from build123d import *

# Parameters (mm, degrees)
SKETCH4_R           = 2
SKETCH4_R_2         = 2.85
SKETCH4_W           = 22
SKETCH4_H           = 32
BOSS_EXTRUDE1_DEPTH = 5
FILLET1_R           = 5
CHAMFER1_SIZE       = 0.5


with BuildPart() as part:
    # Sketch4 → Boss-Extrude1 (new, symmetric)
    with BuildSketch(Plane.XY):
        with BuildLine():
            ThreePointArc((69.282032303, -10), (0, 70), (-69.282032303, -10))
            Line((-69.282032303, -10), (-35, 9.792740578))
            Line((-35, 9.792740578), (-35, -55))
            Line((-35, -55), (-35, -65))
            Line((-35, -65), (-15, -105))
            Line((-15, -105), (-7.5, -105))
            Line((-7.5, -105), (-7.5, -90))
            Line((-7.5, -90), (7.5, -90))
            Line((7.5, -90), (7.5, -105))
            Line((7.5, -105), (15, -105))
            Line((15, -105), (35, -65))
            Line((35, -65), (35, 9.792740578))
            Line((35, 9.792740578), (69.282032303, -10))
        make_face()
        with Locations((-8.75, -87)):
            Circle(SKETCH4_R, mode=Mode.SUBTRACT)
        with Locations((-25, -45)):
            Circle(SKETCH4_R_2, mode=Mode.SUBTRACT)
        with Locations((8.75, -87)):
            Circle(SKETCH4_R, mode=Mode.SUBTRACT)
        with Locations((25, -45)):
            Circle(SKETCH4_R_2, mode=Mode.SUBTRACT)
        with BuildLine():
            Line((25, -32.5), (-25, -32.5))
            ThreePointArc((-25, -32.5), (-27.5, -30), (-25, -27.5))
            Line((-25, -27.5), (25, -27.5))
            ThreePointArc((25, -27.5), (27.5, -30), (25, -32.5))
        make_face(mode=Mode.SUBTRACT)
        with Locations((-18, 0)):
            Circle(SKETCH4_R_2, mode=Mode.SUBTRACT)
        with BuildLine():
            Line((-30, 24.226497308), (-59.572090597, 7.153042841))
            ThreePointArc((-59.572090597, 7.153042841), (-50.077338732, 33.04935923), (-30, 51.961524227))
            Line((-30, 51.961524227), (-30, 24.226497308))
        make_face(mode=Mode.SUBTRACT)
        with Locations((-22, 30)):
            Circle(SKETCH4_R_2, mode=Mode.SUBTRACT)
        with Locations((0, 46)):
            Rectangle(SKETCH4_W, SKETCH4_H, mode=Mode.SUBTRACT)
        with Locations((18, 0)):
            Circle(SKETCH4_R_2, mode=Mode.SUBTRACT)
        with BuildLine():
            Line((25, 12.5), (-25, 12.5))
            ThreePointArc((-25, 12.5), (-27.5, 15), (-25, 17.5))
            Line((-25, 17.5), (25, 17.5))
            ThreePointArc((25, 17.5), (27.5, 15), (25, 12.5))
        make_face(mode=Mode.SUBTRACT)
        with Locations((22, 30)):
            Circle(SKETCH4_R_2, mode=Mode.SUBTRACT)
        with BuildLine():
            Line((59.572090597, 7.153042841), (30, 24.226497308))
            Line((30, 24.226497308), (30, 51.961524227))
            ThreePointArc((30, 51.961524227), (50.077338732, 33.04935923), (59.572090597, 7.153042841))
        make_face(mode=Mode.SUBTRACT)
    extrude(amount=BOSS_EXTRUDE1_DEPTH, both=True)

    # Fillet1
    # the kernel refuses this fillet: 5 mm, written as the material it adds along each edge
    with BuildSketch(Plane(origin=(59.572090597, 7.153042841, -5), x_dir=(-0.8660254037844397, 0.49999999999999806, 0), z_dir=(0, 0, 1))) as fillet1_piece_1:
        with BuildLine():
            CenterArc((11.332313176, -5), FILLET1_R, 90, 138.168098297)
            ThreePointArc((7.997575975, -8.725523829), (3.783101322, -4.560454399), (0, 0))
            Line((0, 0), (11.332313176, 0))
        make_face()
    extrude(amount=10)
    with BuildSketch(Plane(origin=(30, 24.226497308, 5), x_dir=(0, 1, 0), z_dir=(0, 0, -1))) as fillet1_piece_2:
        with BuildLine():
            CenterArc((FILLET1_R * 0.57735026919, FILLET1_R), FILLET1_R, 210, 60)
            Line((-FILLET1_R * 0.288675134595, FILLET1_R * 0.5), (0, 0))
            Line((0, 0), (FILLET1_R * 0.57735026919, 0))
        make_face()
    extrude(amount=10)
    with BuildSketch(Plane(origin=(30, 51.961524227, -5), x_dir=(0, -1, 0), z_dir=(0, 0, 1))) as fillet1_piece_3:
        with BuildLine():
            CenterArc((9.535117356, 5), FILLET1_R, 140.478803641, 129.521196359)
            ThreePointArc((5.678171277, 8.181818182), (2.669034839, 4.208924127), (0, 0))
            Line((0, 0), (9.535117356, 0))
        make_face()
    extrude(amount=10)
    with BuildSketch(Plane(origin=(-59.572090597, 7.153042841, 5), x_dir=(0.2165677144201491, 0.9762675991094004, 0), z_dir=(0, 0, -1))) as fillet1_piece_4:
        with BuildLine():
            CenterArc((11.343039457, 4.975618333), FILLET1_R, 137.492482071, 138.168098297)
            Line((7.657096034, 8.354053043), (0, 0))
            ThreePointArc((0, 0), (5.918107543, -0.29258), (11.836215086, 0))
        make_face()
    extrude(amount=10)
    with BuildSketch(Plane(origin=(-30, 24.226497308, -5), x_dir=(-0.8660254037844397, -0.49999999999999795, 0), z_dir=(0, 0, 1))) as fillet1_piece_5:
        with BuildLine():
            CenterArc((FILLET1_R * 0.57735026919, -FILLET1_R), FILLET1_R, 90, 60)
            Line((-FILLET1_R * 0.288675134595, -FILLET1_R * 0.5), (0, 0))
            Line((0, 0), (FILLET1_R * 0.57735026919, 0))
        make_face()
    extrude(amount=10)
    with BuildSketch(Plane(origin=(-30, 51.961524227, -5), x_dir=(-0.8215414898046486, -0.5701487354450225, 0), z_dir=(0, 0, 1))) as fillet1_piece_6:
        with BuildLine():
            CenterArc((9.544142552, 4.982750841), FILLET1_R, 145.239401821, 129.521196359)
            Line((5.436435103, 7.833494518), (0, 0))
            ThreePointArc((0, 0), (4.979552636, -0.206989911), (9.959105271, 0))
        make_face()
    extrude(amount=10)
    with BuildSketch(Plane(origin=(35, 9.792740578, -5), x_dir=(0.8660254037844399, -0.49999999999999795, 0), z_dir=(0, 0, 1)), Plane(origin=(-35, 9.792740578, -5), x_dir=(0, -1, 0), z_dir=(0, 0, 1))) as fillet1_piece_7:
        with BuildLine():
            CenterArc((FILLET1_R * 1.73205080757, -FILLET1_R), FILLET1_R, 90, 120)
            Line((FILLET1_R * 0.866025403784, -FILLET1_R * 1.5), (0, 0))
            Line((0, 0), (FILLET1_R * 1.73205080757, 0))
        make_face()
    extrude(amount=10)
    with BuildSketch(Plane(origin=(7.5, -90, 5), x_dir=(0, -1, 0), z_dir=(0, 0, -1)), Plane(origin=(-7.5, -90, 5), x_dir=(1, 0, 0), z_dir=(0, 0, -1))) as fillet1_piece_8:
        with BuildLine():
            CenterArc((FILLET1_R, FILLET1_R), FILLET1_R, 180, 90)
            Line((0, FILLET1_R), (0, 0))
            Line((0, 0), (FILLET1_R, 0))
        make_face()
    extrude(amount=10)
    # the kernel refuses this fillet: 5 mm, written as the material it takes off along each edge
    with BuildSketch(Plane(origin=(-69.282032303, -10, -25.386938297), x_dir=(-0.08496362878818808, 0.9963840533565073, 0), z_dir=(0, 0, 1))) as fillet1_2_piece_1:
        with BuildLine():
            CenterArc((7.863533343, -4.991510604), FILLET1_R, 86.660722685, 118.465343928)
            Line((3.33665476, -7.114567433), (0, 0))
            ThreePointArc((0, 0), (4.077387659, 0.118851542), (8.154775319, 0))
        make_face()
    extrude(amount=50.773876593, mode=Mode.SUBTRACT)
    with BuildSketch(Plane(origin=(69.282032303, -10, -25.386938297), x_dir=(-0.8660254037844397, 0.4999999999999982, 0), z_dir=(0, 0, 1))) as fillet1_2_piece_2:
        with BuildLine():
            CenterArc((7.858138122, -5), FILLET1_R, 90, 118.465343928)
            ThreePointArc((3.462610285, -7.383135547), (1.623699843, -3.742033489), (0, 0))
            Line((0, 0), (7.858138122, 0))
        make_face()
    extrude(amount=50.773876593, mode=Mode.SUBTRACT)
    with BuildSketch(Plane(origin=(15, -105, -12.725424859), x_dir=(-1, 0, 0), z_dir=(0, 0, 1)), Plane(origin=(-15, -105, -12.725424859), x_dir=(-0.4472135954999598, 0.894427190999915, 0), z_dir=(0, 0, 1))) as fillet1_2_piece_3:
        with BuildLine():
            CenterArc((FILLET1_R * 0.61803398875, -FILLET1_R), FILLET1_R, 90, 63.434948823)
            Line((-FILLET1_R * 0.27639320225, -FILLET1_R * 0.5527864045), (0, 0))
            Line((0, 0), (FILLET1_R * 0.61803398875, 0))
        make_face()
    extrude(amount=25.450849719, mode=Mode.SUBTRACT)
    with BuildSketch(Plane(origin=(7.5, -105, -17.5), x_dir=(0, 1, 0), z_dir=(0, 0, 1))) as fillet1_2_piece_4:
        with BuildLine():
            CenterArc((FILLET1_R, -FILLET1_R), FILLET1_R, 90, 90)
            Line((0, -FILLET1_R), (0, 0))
            Line((0, 0), (FILLET1_R, 0))
        make_face()
    extrude(amount=35, mode=Mode.SUBTRACT)
    with BuildSketch(Plane(origin=(-7.5, -105, 17.5), x_dir=(-1, 0, 0), z_dir=(0, 0, -1))) as fillet1_2_piece_5:
        with BuildLine():
            CenterArc((FILLET1_R, FILLET1_R), FILLET1_R, 180, 90)
            Line((0, FILLET1_R), (0, 0))
            Line((0, 0), (FILLET1_R, 0))
        make_face()
    extrude(amount=35, mode=Mode.SUBTRACT)

    # Chamfer1
    chamfer1_edges = [part.edges().sort_by_distance(p)[0] for p in [
        (22.15, -45, 5),
        (19.15, 30, 5),
        (15.15, 0, 5),
        (6.75, -87, 5),
        (-10.75, -87, 5),
        (-24.85, 30, 5),
        (-20.85, 0, 5),
        (-27.85, -45, 5),
    ]]
    chamfer(chamfer1_edges, length=CHAMFER1_SIZE)


solid = part.part
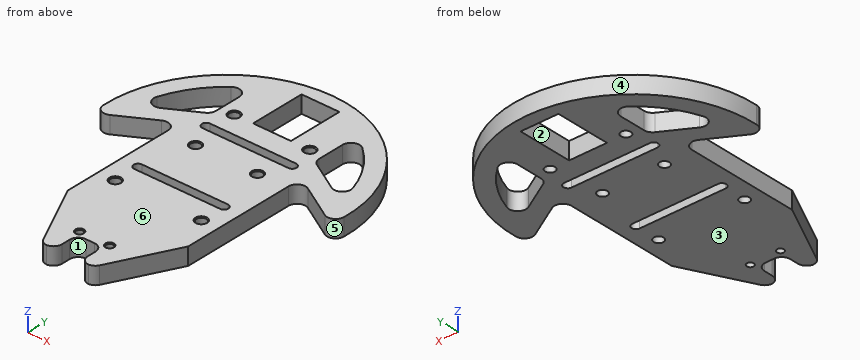
Source: CAD feature listing. Evaluate the final solid. Frame: model axes, mm. Face numbers are marked on the shaded views. A direction names the side the tool comes from. Coordinates: 2 decimals unless noted, no trailing zeros. Write each loop counter-clockwise with the first axis right and the second up, starting at its lowest first coordinate (ties: lowest second). Pieces come first, ordered by that corner, then holes. Notation, with made-up numbers: M 87.25,-18.75 L 94.25,-18.75 A20 ccw 94.25,0.25 Z; hole C -39,63.25 d1. An arc over 180 degrees is marked long. Use a Markdown table: item, result.
1) Ray query, L1, parallel to Y at x = -15, z = -1; L2, parallel to Y at x = -18, z = 1; L3, parallel to X at y = 34, z = -2.25. Return the intervals inside material, ascending.
Conclusion:
| item | result |
|---|---|
| L1 | y = -103.93 to -32.5, -27.5 to 12.5, 17.5 to 68.37 |
| L2 | y = -99 to -32.5, -27.5 to -2.85, 2.85 to 12.5, 17.5 to 67.65 |
| L3 | x = -61.19 to -49.44, -30 to -11, 11 to 30, 49.44 to 61.19 |
2) Section A-A, the plane y = -87. Output: boundary loops of the cut face in (x, z).
Conclusion:
| item | result |
|---|---|
| outline | M -24,-5 L -10.75,-5 L -10.75,4.5 L -11.25,5 L -24,5 Z; M -6.75,-5 L 6.75,-5 L 6.75,4.5 L 6.25,5 L -6.25,5 L -6.75,4.5 Z; M 10.75,-5 L 24,-5 L 24,5 L 11.25,5 L 10.75,4.5 Z |
3) Section D-D, the plane x = -45. Output: boundary loops of the cut face in (y, z).
Conclusion:
| item | result |
|---|---|
| outline | M 4.02,-5 L 15.57,-5 L 15.57,5 L 4.02,5 Z; M 39.69,-5 L 53.62,-5 L 53.62,5 L 39.69,5 Z |
4) Section B-B, the plane x = 0. Output: boundary loops of the cut face in (y, z).
Conclusion:
| item | result |
|---|---|
| outline | M -90,-5 L -32.5,-5 L -32.5,5 L -90,5 Z; M -27.5,-5 L 12.5,-5 L 12.5,5 L -27.5,5 Z; M 17.5,-5 L 30,-5 L 30,5 L 17.5,5 Z; M 62,-5 L 70,-5 L 70,5 L 62,5 Z |
5) Reachability of the marked faces 1, 2 and 3 from +Z, -Z, +X, -X, +Y, -Y: full face, straight path, thin tool, end or side. Return the list, or none.
Conclusion:
| item | result |
|---|---|
| face 1 | +Z, -Z, -Y |
| face 2 | +Z, -Z |
| face 3 | -Z, +X, -X, +Y, -Y |
6) Mould query, pull axis X, two halves, no side actions, for the marked faces 4, 5 and 6. Classes: pulls with the +X half, pulls with the -X half, needs draft (parallel to the pull), parting line crosses it, or undercut.
Conclusion:
| item | result |
|---|---|
| face 4 | parting line crosses it |
| face 5 | undercut |
| face 6 | needs draft |
7) First-contact query: pin 1 Ø7.5 at (x, y) = (25, -45) entering from +Z; pin 2 Ø5 at (y, z) = (-23.5, 0.5) entering from +X; pin 3 Ø5.5 at (y, z) = (-97.5, 1.5) entering from -X (3 decimals); pin 4 Ø4 at (x, z) = (45, 2) entering from +Y. Flat tips, straight axial feed; report the tip coordinate or a pass-through.
Conclusion:
| item | result |
|---|---|
| pin 1 | stops at z = 5 |
| pin 2 | stops at x = 35 |
| pin 3 | stops at x = -20.125 |
| pin 4 | stops at y = 55.24 |
8) Section C-C, the plane y = 15. Output: boundary loops of the cut face in (x, z).
Conclusion:
| item | result |
|---|---|
| outline | M -68.37,-5 L -56.77,-5 L -56.77,5 L -68.37,5 Z; M -45.98,-5 L -27.5,-5 L -27.5,5 L -45.98,5 Z; M 27.5,-5 L 45.98,-5 L 45.98,5 L 27.5,5 Z; M 56.77,-5 L 68.37,-5 L 68.37,5 L 56.77,5 Z |
